Design review of the part shown in the three views and the two pictorial views. Dimensions are in mm from the part's minimum x, y and z. A direction names the side the tool comes from. Give positions to 0.01 mm unless a question says otherwise; leave off trailing zeros. Order: outer loops, then holes, each group sorted by start corner. A loop starts at its lowest first (then second) coordinate and runs counter-clockwise, first axis right, second up. Notation, with made-up numbers: (65, 58.5) - (109, 58.5) arc R24 cw to (109, 81.5) - close; hole circle Ø1 at (-39.5, -5.75). An arc over 180 degrees is marked (long way). Put each result on its own line as item: value.
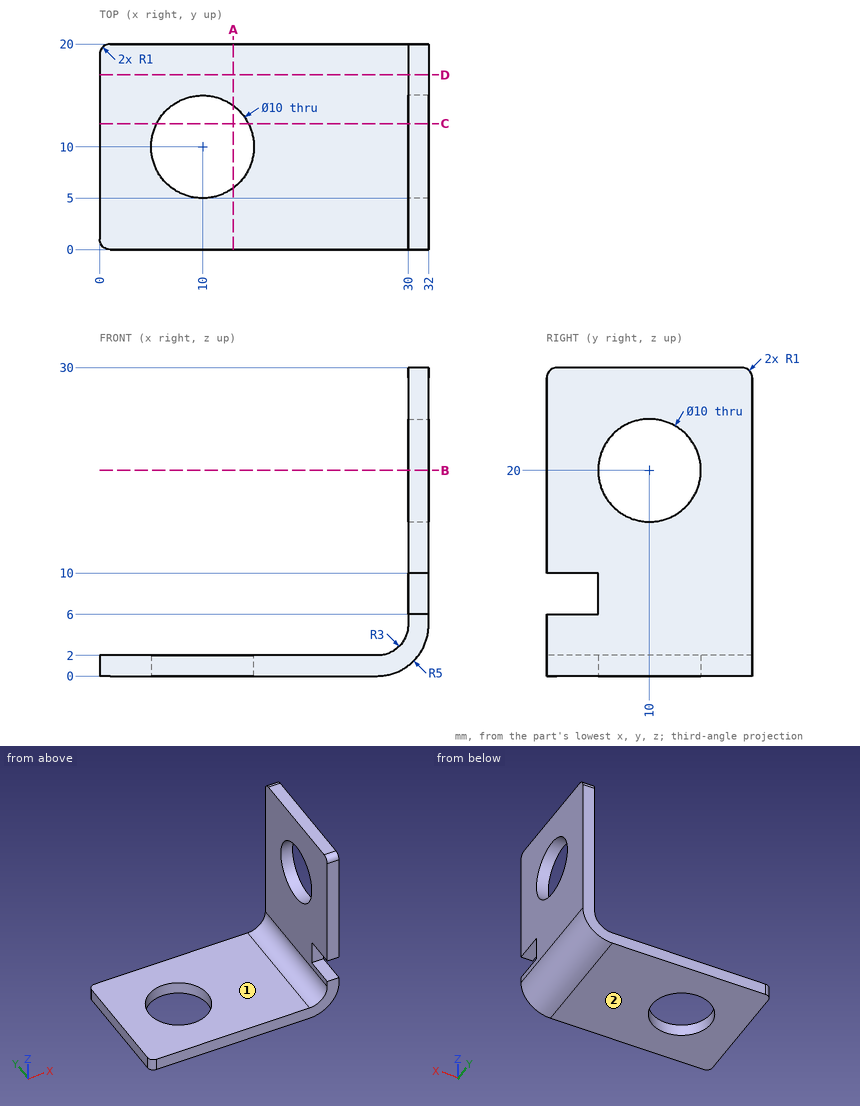
(1) Take a section at A-A, the plane x = 13. Write out the cut boundary in (y, z).
The answers:
outline: (0, 0) - (6, 0) - (6, 2) - (0, 2) - close; (14, 0) - (20, 0) - (20, 2) - (14, 2) - close
(2) Clearance check with flat-ended pins moving along their axes: pin 1 Ø1 at (x, y) = (12.5, 4) entering from +Z; pin 2 Ø2 at (y, z) = (2, 18.5) entering from -X; pin 3 Ø12 at (x, z) = (23, 16.5) entering from -Y; pin 4 Ø1 at (x, y) = (31, 3) entering from -Z. State where each tip first meets the part, or that it passes through.
The answers:
pin 1: z = 2
pin 2: x = 30
pin 3: through
pin 4: z = 1.43
(3) For the marked faces 1 and 2, list the 3-axis set-ups (+Z, -Z, +X, -X, +Y, -Y) from which the entire face can be reached by the end or side of a thin tool; tool diameter is ignored.
The answers:
face 1: +Z, -X, +Y, -Y
face 2: -Z, +X, -X, +Y, -Y
(4) Take a section at C-C, the plane y = 12.25. Write out the cut boundary in (x, z), then the cut area to 3 significant figures.
The answers:
outline: (0, 0) - (5.53, 0) - (5.53, 2) - (0, 2) - close; (14.47, 0) - (27, 0) arc R5 ccw to (32, 5) - (32, 15.53) - (30, 15.53) - (30, 5) arc R3 cw to (27, 2) - (14.47, 2) - close; (30, 24.47) - (32, 24.47) - (32, 30) - (30, 30) - close
area: 80.8 mm^2
(5) Take a section at B-B, the plane z = 20. Write out the cut boundary in (x, y).
The answers:
outline: (30, 0) - (32, 0) - (32, 5) - (30, 5) - close; (30, 15) - (32, 15) - (32, 20) - (30, 20) - close
(6) Wall thickness on L1, parallel to Y at x = 10, z = 0.9; L2, parallel to Z at x = 12.5, y = 2.25; L3, parallel to X at y = 6, z = 7.5: over which ranges is each line inside the solid? List them lowest first.
The answers:
L1: 0 to 5, 15 to 20
L2: 0 to 2
L3: 30 to 32
(7) Take a section at D-D, the plane y = 17. Write out the cut boundary in (x, z).
The answers:
outline: (0, 0) - (27, 0) arc R5 ccw to (32, 5) - (32, 30) - (30, 30) - (30, 5) arc R3 cw to (27, 2) - (0, 2) - close
